Can you work these out from the drawing? Everything is in mm from the part's minimum corner. A direction names the side the tool comes from. Give positions to 0.01 mm unless a question says otherwise; leave off trailing zeros. Loops run counter-clockwise (first coordinate to the right, second up) from the corner with the lowest first, then second, coordinate; pieces in that order, holes last. Notation, with made-up numbers: (34, 52.25) - (41, 52.25) arc R14 ccw to (41, 58.25) - close; hole circle Ø3 at (-10, 75). An arc over 180 degrees is marked (long way). Answer in a Markdown table with one row per item.
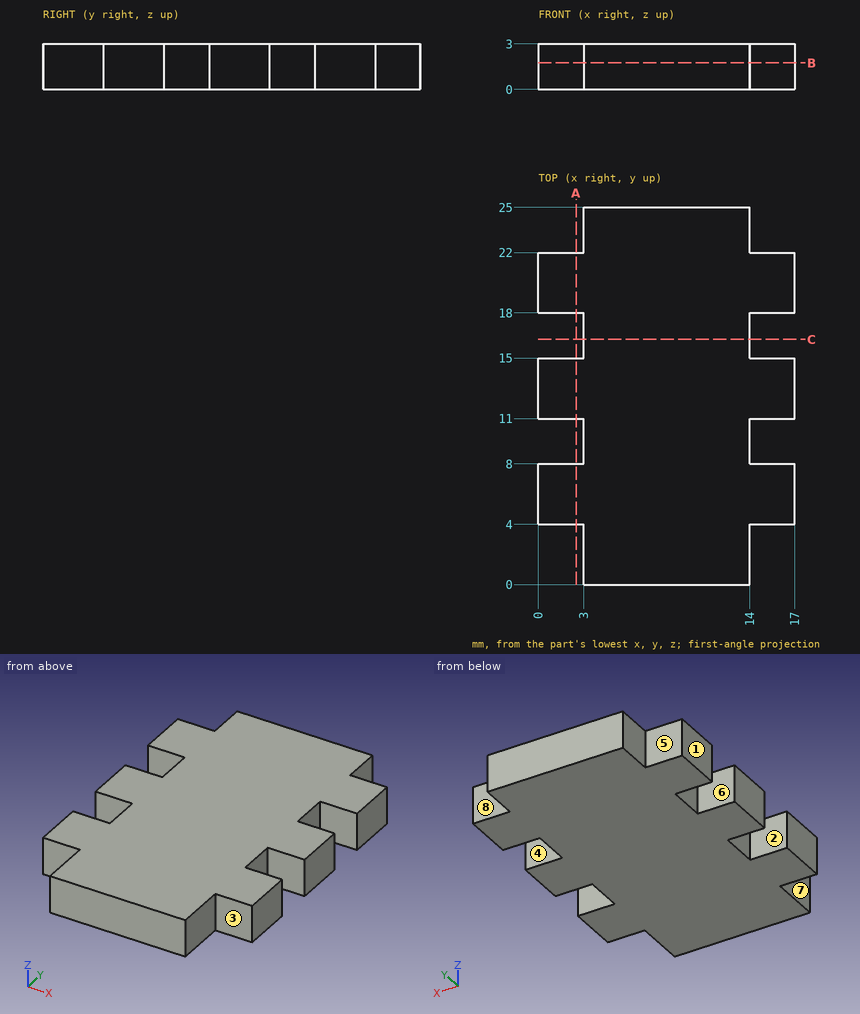
Q1. Imagine slicing it at C-C, the plane y = 16.25. Write out the boundary of the cut face in (x, z).
Checked values:
| item | result |
|---|---|
| outline | (3, 0) - (14, 0) - (14, 3) - (3, 3) - close |
Q2. On a 3-axis mill with a long thin cutter (end or side, diameter ignored), from which of +Z, -Z, +X, -X, +Y, -Y can I reach the whole of each face in a straight line? I mean the marked faces 4, 5, 6, 7 and 8. Say none if no direction works.
Checked values:
| item | result |
|---|---|
| face 4 | +Z, -Z, +X |
| face 5 | +Z, -Z, -X, +Y |
| face 6 | +Z, -Z, -X |
| face 7 | +Z, -Z, -X, -Y |
| face 8 | +Z, -Z, +X, +Y |
Q3. For pin 1 (0.9 mm diameter, centred on x = 1, z = 1, fed in from -Y); pin 2 (1.5 mm diameter, centred on y = 2.5, z = 0.5, fed in from +X); pin 3 (6 mm diameter, centred on x = 12.5, y = 6.5, fed in from -Z); pin 4 (1.5 mm diameter, centred on y = 23.5, z = 1.5, fed in from -X), each with a flat end and sliding along its axis, tell me the tip position at first contact or that it passes through.
Checked values:
| item | result |
|---|---|
| pin 1 | stops at y = 4 |
| pin 2 | stops at x = 14 |
| pin 3 | stops at z = 0 |
| pin 4 | stops at x = 3 |
Q4. Imagine slicing it at B-B, the plane z = 1.75. Write out the boundary of the cut face in (x, y).
Checked values:
| item | result |
|---|---|
| outline | (0, 4) - (3, 4) - (3, 0) - (14, 0) - (14, 4) - (17, 4) - (17, 8) - (14, 8) - (14, 11) - (17, 11) - (17, 15) - (14, 15) - (14, 18) - (17, 18) - (17, 22) - (14, 22) - (14, 25) - (3, 25) - (3, 22) - (0, 22) - (0, 18) - (3, 18) - (3, 15) - (0, 15) - (0, 11) - (3, 11) - (3, 8) - (0, 8) - close |
Q5. If I drill on line 1 (Y direction, x = 14.75, z = 0.85); line 2 (X direction, y = 9, z = 2.75), over which ranges is the centre line in solid material (lowest first)? Write a range as [from, to].
Checked values:
| item | result |
|---|---|
| line 1 | y = [4, 8], [11, 15], [18, 22] |
| line 2 | x = [3, 14] |
Q6. If we mould it in two halves opening along Y, with no side actions, what happens to the marked faces 1, 2 and 3? For each: released by +Y, released by -Y, zero draft, split by the parting line, or undercut.
Checked values:
| item | result |
|---|---|
| face 1 | zero draft |
| face 2 | undercut |
| face 3 | released by -Y |
Q7. Imagine slicing it at A-A, the plane x = 2.5. Write out the boundary of the cut face in (y, z), and give its area (3 significant figures).
Checked values:
| item | result |
|---|---|
| outline | (4, 0) - (8, 0) - (8, 3) - (4, 3) - close; (11, 0) - (15, 0) - (15, 3) - (11, 3) - close; (18, 0) - (22, 0) - (22, 3) - (18, 3) - close |
| area | 36.0 mm² |
